```python
from build123d import *

# Parameters (mm, degrees)
CUT_EXTRUDE2_DEPTH = 7
CIRPATTERN1_COUNT  = 4


with BuildPart() as part:
    # Sketch2 → Revolve1 (revolve)
    with BuildSketch(Plane(origin=(0, 0, 0), x_dir=(1, 0, 0), z_dir=(0, 1, 0))):
        with BuildLine():
            Line((-50, -80), (-50, -70))
            Line((-50, -70), (-40, -70))
            Line((-40, -70), (-40, -30))
            Line((-40, -30), (-36, -30))
            Line((-36, -30), (-32, -70))
            Line((-32, -70), (-16, -70))
            Line((-16, -70), (-6, 0))
            Line((-6, 0), (0, 0))
            Line((0, 0), (0, -20))
            Line((0, -20), (-2, -20))
            Line((-2, -20), (-2, -60))
            Line((-2, -60), (0, -60))
            Line((0, -60), (0, -80))
            Line((0, -80), (-6, -80))
            Line((-6, -80), (-6, -78))
            ThreePointArc((-6, -78), (-6.292893219, -77.292893219), (-7, -77))
            Line((-7, -77), (-40, -77))
            ThreePointArc((-40, -77), (-40.707106781, -77.292893219), (-41, -78))
            Line((-41, -78), (-41, -80))
            Line((-41, -80), (-50, -80))
        make_face()
    revolve(axis=Axis((10, 0, 0), (0, 0, 1)))

    # Sketch3 → Cut-Extrude2 (cut)
    with BuildSketch(Plane(origin=(0, 0, 30), x_dir=(-1, 0, 0), z_dir=(0, 0, -1))):
        with BuildLine():
            Line((31.231056256, -8), (39.355850717, -8))
            ThreePointArc((39.355850717, -8), (40, 0), (39.355850717, 8))
            Line((39.355850717, 8), (31.231056256, 8))
            ThreePointArc((31.231056256, 8), (32, 0), (31.231056256, -8))
        make_face()
    cut_extrude2 = extrude(amount=-CUT_EXTRUDE2_DEPTH, mode=Mode.SUBTRACT)

    # CirPattern1: Cut-Extrude2 ×4 about axis
    cirpattern1_axis = Axis((10, 0, 0), (0, 0, 1))
    for i in range(1, CIRPATTERN1_COUNT):
        add(cut_extrude2.rotate(cirpattern1_axis, i * 360 / CIRPATTERN1_COUNT), mode=Mode.SUBTRACT)


solid = part.part
```
Here's how the part is built. I have some questions about the finished solid (model axes, mm). A direction names the side the tool comes from. Round coordinates to 2 decimals unless told otherwise and drop trailing zeros. Loops run counter-clockwise (first coordinate to the right, second up) from the corner with the lowest first, then second, coordinate; pieces in that order, holes last.
1. Suppose I cut it at B-B, the plane z = 22. Please give me the cut outline in (x, y).
Answers:
outline: circle Ø38.29 at (10, 0); hole circle Ø24 at (10, 0)
2. Suppose I cut it at C-C, the plane z = 44.5. Please give me the cut outline in (x, y).
Answers:
outline: circle Ø100 at (10, 0); circle Ø44.71 at (10, 0); hole circle Ø89.1 at (10, 0); hole circle Ø24 at (10, 0)
3. Suppose I cut it at A-A, the plane z = 54. Please give me the cut outline in (x, y), and give its area (3 significant figures).
Answers:
outline: circle Ø100 at (10, 0); circle Ø47.43 at (10, 0); hole circle Ø87.2 at (10, 0); hole circle Ø24 at (10, 0)
area: 3,200 mm2
4. For faces 1 (the face through (10, 47, 37)), 2 (the face through (-37, -8, 33)), 3 (the face through (2, -47, 33)), 4 (the face through (50.472, 31.033, 79.014)), which set-ups out of +Z, -Z, +X, -X, +Y, -Y let a thin tool reach every point of the face, with its end or its side?
Answers:
face 1: -Z, +Y
face 2: -Z, -X
face 3: -Z, -Y
face 4: +Z
5. Will these pins go through, and if not, where does the flat tip stop? pin 1 (5 mm diameter, centred on x = -36, z = 33.5, fed in from +Y); pin 2 (5 mm diameter, centred on x = -18, y = 41.5, fed in from -Z); pin 3 (3 mm diameter, centred on y = -4.5, z = 29.5, fed in from -X); pin 4 (18 mm diameter, centred on x = 10, y = 0, fed in from +Z).
Answers:
pin 1: stops at y = 24.65
pin 2: stops at z = 30
pin 3: stops at x = -10.07
pin 4: passes through
6. If I drill on probe 1 along X at (y, z) = (0, 79); probe 2 along X at (y, z) = (0, 67); probe 3 along Y at (x, z) = (12, 67), over which ranges is the centre line in solid material (lowest first)?
Answers:
probe 1: x = -50 to -41, -6 to 0, 20 to 26, 61 to 70
probe 2: x = -40 to -32.3, -15.57 to 0, 20 to 35.57, 52.3 to 60
probe 3: y = -49.96 to -42.25, -25.49 to -9.8, 9.8 to 25.49, 42.25 to 49.96
7. Thinking about a two-plate mould opening in X: for faces 5 (the face through (26.609, 12.736, 34.51)), 6 (the face through (-47.23, -18.02, 74.93)), 7 (the face through (-37, 0, 37)), which applies, released by +X, released by -X, zero draft, split by the parting line, or undercut?
Answers:
face 5: undercut
face 6: split by the parting line
face 7: zero draft
